Geometry check sheet. Reference: the model listing, model coordinates, mm. A direction names the side the tool comes from. Coordinates: 2 decimals unless noted, no trailing zeros. Write each loop counter-clockwise with the first axis right and the second up, starting at its lowest first coordinate (ties: lowest second). Pieces come first, ordered by that corner, then holes. Notation, with made-up numbers: M -5,25.25 L 36,25.25 A19 cw 36,43.25 Z; hole C -35.75,30.25 d11. An arc over 180 degrees is marked long. Write item = value, one per line. Start each with the question number.
```python
from build123d import *

# Parameters (mm, degrees)
SKETCH_1_W          = 199
SKETCH_1_H          = 99
EXTRUDE_1_DEPTH     = 40
SKETCH_3_W          = 17.5
SKETCH_3_H          = 97.5
CUT_EXTRUDE_2_DEPTH = 30
SKETCH_6_W          = 5
SKETCH_6_H          = 38.2
CUT_EXTRUDE_5_DEPTH = 97.2
SKETCH_7_W          = 17.5
SKETCH_7_H          = 9
CUT_EXTRUDE_6_DEPTH = 8.2
SKETCH_2_R          = 2
CUT_EXTRUDE_1_DEPTH = 10
SKETCH_4_R          = 1.5
CUT_EXTRUDE_3_DEPTH = 10
SKETCH_5_R          = 1.6
CUT_EXTRUDE_4_DEPTH = 10
SKETCH_8_R          = 1.5
CUT_EXTRUDE_7_DEPTH = 119.11223476


with BuildPart() as part:
    # 草图1 → 拉伸1 (new body)
    with BuildSketch(Plane.XY):
        Rectangle(SKETCH_1_W, SKETCH_1_H)
    extrude(amount=EXTRUDE_1_DEPTH)

    # 草图3 → 切除-拉伸2 (cut)
    with BuildSketch(Plane.XY.offset(40)):
        with Locations((-90.75, 0.75)):
            Rectangle(SKETCH_3_W, SKETCH_3_H)
    extrude(amount=-CUT_EXTRUDE_2_DEPTH, mode=Mode.SUBTRACT)

    # 草图6 → 切除-拉伸5 (cut)
    with BuildSketch(Plane(origin=(0, 49.5, 0), x_dir=(-1, 0, 0), z_dir=(0, 1, 0))):
        with Locations((-97, 20.9)):
            Rectangle(SKETCH_6_W, SKETCH_6_H)
    extrude(amount=-CUT_EXTRUDE_5_DEPTH, mode=Mode.SUBTRACT)

    # 草图7 → 切除-拉伸6 (cut)
    with BuildSketch(Plane.XY.offset(10)):
        with Locations((-90.75, -43.5)):
            Rectangle(SKETCH_7_W, SKETCH_7_H)
    extrude(amount=-CUT_EXTRUDE_6_DEPTH, mode=Mode.SUBTRACT)

    # 草图2 → 切除-拉伸1 (cut)
    with BuildSketch(Plane.XY):
        with Locations((-41.5, 39.8)):
            Circle(SKETCH_2_R)
        with Locations((78.5, 39.8)):
            Circle(SKETCH_2_R)
        with Locations((-41.5, -40.2)):
            Circle(SKETCH_2_R)
        with Locations((78.5, -40.2)):
            Circle(SKETCH_2_R)
    extrude(amount=CUT_EXTRUDE_1_DEPTH, mode=Mode.SUBTRACT)

    # 草图4 → 切除-拉伸3 (cut)
    with BuildSketch(Plane.XZ.offset(49.5)):
        with Locations(Location((-79.5, 20, 0), (0, 0, 270))):
            Circle(SKETCH_4_R)
        with Locations(Location((77.5, 12.5, 0), (0, 0, 270))):
            Circle(SKETCH_4_R)
        with Locations(Location((77.5, 30.5, 0), (0, 0, 270))):
            Circle(SKETCH_4_R)
    extrude(amount=-CUT_EXTRUDE_3_DEPTH, mode=Mode.SUBTRACT)

    # 草图5 → 切除-拉伸4 (cut)
    with BuildSketch(Plane.XZ.offset(49.5)):
        with Locations(Location((-93, 29, 0), (0, 0, 270))):
            Circle(SKETCH_5_R)
        with BuildLine():
            Line((99.5, 34.5), (99.5, 31.3))
            Line((99.5, 31.3), (98.2, 31.3))
            ThreePointArc((98.2, 31.3), (96.6, 32.9), (98.2, 34.5))
            Line((98.2, 34.5), (99.5, 34.5))
        make_face()
    extrude(amount=-CUT_EXTRUDE_4_DEPTH, mode=Mode.SUBTRACT)

    # 草图8 → 切除-拉伸7 (cut, through all)
    with BuildSketch(Plane(origin=(0, 0, 0), x_dir=(-1, 0, 0), z_dir=(0, 0, -1))):
        with Locations((-96, 41.8)):
            Circle(SKETCH_8_R)
        with Locations((-96, -43.7)):
            Circle(SKETCH_8_R)
        with Locations((95, -43.7)):
            Circle(SKETCH_8_R)
        with Locations(Location((95, 41.8, 0), (0, 0, 180))):
            Circle(SKETCH_8_R)
    extrude(amount=-CUT_EXTRUDE_7_DEPTH, mode=Mode.SUBTRACT)


solid = part.part
```
Q1. Gauge pin test, flat ends, axial feed: pin 1 (2.5 mm diameter, centred on x = -95, y = 41.8, fed in from -Z); pin 2 (5 mm diameter, centred on x = -93, z = 23.5, fed in from +Y); pin 3 (1.5 mm diameter, centred on x = 78, z = 30, fed in from -Y); pin 4 (1.2 mm diameter, centred on x = 78, y = -39.5, fed in from -Z). Record the tip position at first contact, or that the pin passes through.
Q2. Scan lines: L1, parallel to Y at x = -41.5, z = 5.75; L2, parallel to Z at x = 77.5, y = -45.5; L3, parallel to X at y = -44, z = 25.5. Record each from-to range of solid material in increasing order.
Q3. Set-up check for faces 5 (the face through (-91, -43, 1.8)), 6 (the face through (-91, 6, 10)), 7 (the face through (-42, -40, 10)), 8 (the face through (97, -47.7, 21)): record each of +Z, -Z, +X, -X, +Y, -Y from which the full face is reachable in a straight line by a thin tool's end or side.
Q4. Draft check along Y on faces 1 (the face through (-99.5, 3, 7)), 2 (the face through (-1, 49.5, 20)), 3 (the face through (-41.76, -38.217, 4.93)), 4 (the face through (-91, -39, 6)). Enter one of: pulls with the +Y half, pulls with the -Y half, needs draft (parallel to the pull), parting line crosses it, or undercut.
Q5. Cross-section at A-A on y = 23.5. Enter the section's corners in (x, z), and give its area (3 significant figures).
Values found:
q1.pin_1 = through
q1.pin_2 = -48
q1.pin_3 = -39.5
q1.pin_4 = 10
q2.L1 = -49.5 to -42.2, -38.2 to 37.8, 41.8 to 49.5
q2.L2 = 0 to 11, 14 to 29, 32 to 40
q2.L3 = -82 to 94.5
q3.face_5 = +Z, -X
q3.face_6 = +Z, -X, +Y
q3.face_7 = -Z
q3.face_8 = +Z, +X, +Y
q4.face_1 = needs draft
q4.face_2 = pulls with the +Y half
q4.face_3 = undercut
q4.face_4 = undercut
q5.outline = M -99.5,0 L 99.5,0 L 99.5,1.8 L 94.5,1.8 L 94.5,40 L -82,40 L -82,10 L -99.5,10 Z
q5.area = 7,240 mm²
